The listing builds one solid part. Answer for the finished solid, in the listing's coordinates (mm). Face numbers are marked on the shaded views. A direction names the side the tool comes from. Give positions to 0.01 mm unless a question says otherwise; leave off trailing zeros. Write each loop counter-clockwise with the first axis right and the second up, starting at its lowest first coordinate (ties: lowest second). Pieces come first, ordered by that corner, then holes. Notation, with made-up numbers: M 16.25,-28.5 L 66.25,-28.5 A7 ccw 66.25,-16.5 Z; hole C 12,69.25 d1. An arc over 180 degrees is marked long. Answer as a JSON object with one key per item and string values.
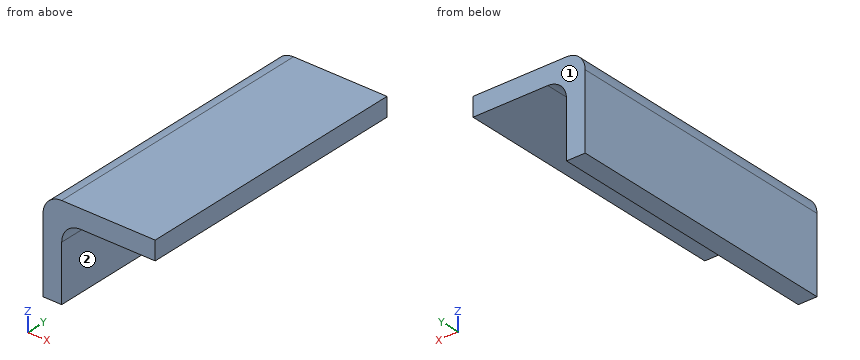
Autodesk Inventor part; units mm, degrees
ref_plane "YZ Plane" through (0, 0, 0) normal (1, 0, 0) x (0, 1, 0)
ref_plane "XZ Plane" through (0, 0, 0) normal (0, 1, 0) x (-1, 0, 0)
ref_plane "XY Plane" through (0, 0, 0) normal (0, 0, 1) x (1, 0, 0)
sketch "Sketch1" plane through (0, 0, 0) normal (0, 1, 0) x (-1, 0, 0)
  line L0 (-2, 0) -> (-2, 0)
  line L1 (-2, -4) -> (-2, -10)
  line L2 (-2, -10) -> (0, -10)
  line L3 (0, -10) -> (0, -2)
  line L4 (-2, 0) -> (-12, 0)
  line L5 (-12, 0) -> (-12, -2)
  line L6 (-12, -2) -> (-4, -2)
  line L7 (-2, -2) -> (-2, 0)
  arc A0 (-2, -4) -> (-4, -2) centre (-4, -4) ccw
  arc A1 (0, -2) -> (-2, 0) centre (-2, -2) ccw
  point P0 (0, 0)
  dimension "d0" = 2
  dimension "d1" = 2
  dimension "d2" = 10
  dimension "d3" = 10
  dimension "d4" = 2
  dimension "d5" = 2
extrude "Extrusion1" add sketch "Sketch1" along normal blind 30
equation "\"d1\" = d0"
properties material "Aluminum 6061"
1. Consider line 1 along Z through (x, y) = (9.25, 12); line 2 along X through (y, z) = (26.75, -6); line 3 along X through (y, z) = (16, -1.5). Determine where each line is inside the solid, lowest interval first.
Verdict:
{"line 1": "z = -2 to 0", "line 2": "x = 0 to 2", "line 3": "x = 0.06 to 12"}
2. For the marked faces 1 and 2, determine the directions among +Z, -Z, +X, -X, +Y, -Y from which every point of the face is accessible in a straight line to the end or side of a thin tool.
Verdict:
{"face 1": "+Z, -Z, +X, -X, +Y", "face 2": "-Z, +X, +Y, -Y"}
3. A cutting plane is placed at B-B, the plane z = -7. Give the vertices of the cut face in (x, y).
Verdict:
{"outline": "M 0,0 L 2,0 L 2,30 L 0,30 Z"}
4. A flat-ended cylindrical pin translates along its axis: pin 1 (1.8 mm diameter, centred on y = 14.5, z = -6, fed in from +X). Find the tip coordinate at first contact, or state that the pin passes through.
Verdict:
{"pin 1": "stops at x = 2"}
5. A cutting plane is placed at A-A, the plane y = 19.25. Give the vertices of the cut face in (x, z).
Verdict:
{"outline": "M 0,-10 L 2,-10 L 2,-4 A2 cw 4,-2 L 12,-2 L 12,0 L 2,0 A2 ccw 0,-2 Z"}
6. A cutting plane is placed at C-C, the plane x = 10. Give the vertices of the cut face in (y, z).
Verdict:
{"outline": "M 0,-2 L 30,-2 L 30,0 L 0,0 Z"}
